Work out the finished part from the listing and answer in its coordinate system (mm). Face numbers are marked on the shaded views. Give positions to 0.01 mm unless a question says otherwise; leave off trailing zeros. Write each loop counter-clockwise with the first axis right and the second up, starting at its lowest first coordinate (ties: lowest second). Pieces come first, ordered by that corner, then holes.
1) Find section B-B (x = -7). Determine the outline of the cut face in (y, z), plus the area to 3 significant figures.
2) Find section C-C (y = 0). Determine the outline of the cut face in (x, z).
3) Given pin 1 Ø3 at (x, y) = (8, 2) entering from +Z; pin 2 Ø1.5 at (x, y) = (41, -1.5) entering from +Z; pin 3 Ø3 at (x, z) = (5, 1.5) entering from +Y; pin 4 Ø5 at (y, z) = (-1.5, 8.5) entering from +X, each flat-ended and moving along its own axis, determine where each tip first touches the part or whether it passes through.
4) Straight lines are drawn through the part: probe 1 along Y at (x, z) = (42, 0); probe 2 along X at (y, z) = (5.05, 0); probe 3 along X at (y, z) = (4.5, 0). For each, find the intervals that lie inside material, in ascending order.
5) Determine the mould class of the marked faces 1, 2 and 3 for opening direction Z: pulls with the +Z half, pulls with the -Z half, needs draft (parallel to the pull), parting line crosses it, or undercut.
6) Find section D-D (x = 41). Determine the outline of the cut face in (y, z), plus the area to 3 significant figures.
```python
from build123d import *

# Parameters (mm, degrees)
CUT_EXTRUDE1_DEPTH      = 28.440845468
CUT_EXTRUDE1_DEPTH_BACK = 28.440845468
SKETCH3_W               = 33
SKETCH3_H               = 8.75
SKETCH4_W               = 0.2
SKETCH4_H               = 1
SKETCH5_R               = 5
BOSS_EXTRUDE1_DEPTH     = 29
CHAMFER1_SIZE           = 1
ESQUISSE1_R             = 4
ENL_V_MAT_EXTRU_1_DEPTH = 10


with BuildPart() as part:
    # Sketch2 → Revolve2 (revolve)
    with BuildSketch(Plane(origin=(0, 0, 0), x_dir=(1, 0, 0), z_dir=(0, 1, 0))):
        with BuildLine():
            Line((7.147970434, 12.037712352), (19, 5))
            Line((19, 5), (19, 0))
            Line((19, 0), (-14, 0))
            ThreePointArc((-14, 0), (-6.925619609, 12.166996056), (7.147970434, 12.037712352))
        make_face()
    revolve(axis=Axis((-39.456415939, 0, 0), (1, 0, 0)))

    # Sketch3 → Cut-Extrude1 (cut, two sides: drawn at the far end of the back side and taken through both)
    with BuildSketch(Plane.XY.offset(-CUT_EXTRUDE1_DEPTH_BACK)):
        with Locations((2.5, 9.625)):
            Rectangle(SKETCH3_W, SKETCH3_H)
        with Locations((2.5, -9.625)):
            Rectangle(SKETCH3_W, SKETCH3_H)
    extrude(amount=CUT_EXTRUDE1_DEPTH + CUT_EXTRUDE1_DEPTH_BACK, mode=Mode.SUBTRACT)

    # Sketch4 → Cut-Revolve1 (revolve, cut)
    with BuildSketch(Plane.XY, mode=Mode.PRIVATE) as cut_revolve1_sk:
        with BuildLine():
            Line((0, 10), (0, -10))
            ThreePointArc((0, -10), (10, 0), (0, 10))
        make_face()
        with Locations((11.1, 4.75)):
            Rectangle(SKETCH4_W, SKETCH4_H)
        with Locations((11.1, -4.75)):
            Rectangle(SKETCH4_W, SKETCH4_H)
    revolve(cut_revolve1_sk.sketch.rotate(Axis((0, 13.975998128, 0), (0, -1, 0)), 90), axis=Axis((0, 13.975998128, 0), (0, -1, 0)), mode=Mode.SUBTRACT)

    # Sketch5 → Boss-Extrude1 (add)
    with BuildSketch(Plane(origin=(19, 0, 0), x_dir=(0, 0, -1), z_dir=(1, 0, 0))):
        with Locations(Location((0, 0, 0), (0, 0, 180))):
            Circle(SKETCH5_R)
    extrude(amount=BOSS_EXTRUDE1_DEPTH)

    # Chamfer1
    chamfer1_edges = [part.edges().sort_by_distance(p)[0] for p in [
        (48, 0, -5),
    ]]
    chamfer(chamfer1_edges, length=CHAMFER1_SIZE)

    # Esquisse1 → Enl_v. mat.-Extru.1 (cut)
    with BuildSketch(Plane(origin=(48, 0, 0), x_dir=(0, 0, -1), z_dir=(1, 0, 0))):
        Circle(ESQUISSE1_R)
    extrude(amount=-ENL_V_MAT_EXTRU_1_DEPTH, mode=Mode.SUBTRACT)


solid = part.part
```
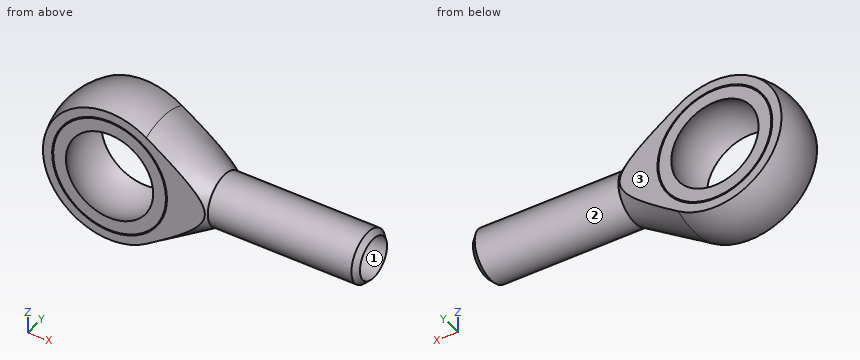
Results:
1. outline: (-5.25, -10.93) arc R12.12 ccw to (5.25, -10.93) - (5.25, -8.74) - (4.25, -8.74) - (4.25, -8.49) - (5.25, -8.49) - (5.25, -4.84) arc R7.14 cw to (-5.25, -4.84) - (-5.25, -8.49) - (-4.25, -8.49) - (-4.25, -8.74) - (-5.25, -8.74) - close; (-5.25, 4.84) arc R7.14 cw to (5.25, 4.84) - (5.25, 8.49) - (4.25, 8.49) - (4.25, 8.74) - (5.25, 8.74) - (5.25, 10.93) arc R12.12 ccw to (-5.25, 10.93) - (-5.25, 8.74) - (-4.25, 8.74) - (-4.25, 8.49) - (-5.25, 8.49) - close
1. area: 110 mm2
2. outline: (7.15, -12.04) - (19, -5) - (47, -5) - (48, -4) - (38, -4) - (38, 4) - (48, 4) - (47, 5) - (19, 5) - (7.15, 12.04) arc R14 ccw (long way) to start; hole circle Ø20 at (0, 0)
3. pin 1: stops at z = 12.27
3. pin 2: stops at z = 4.94
3. pin 3: passes through
3. pin 4: stops at x = 17.09
4. probe 1: y = -5 to -4, 4 to 5
4. probe 2: x = -13.06 to -11.2, -11 to -8.63, 8.63 to 11, 11.2 to 18.92
4. probe 3: x = -13.26 to -11.2, -11 to -8.93, 8.93 to 11, 11.2 to 47.5
5. face 1: undercut
5. face 2: parting line crosses it
5. face 3: needs draft
6. outline: circle Ø10 at (0, 0); hole circle Ø8 at (0, 0)
6. area: 28.3 mm2
